```python
from build123d import *

# Parameters (mm, degrees)
F1_DEPTH      = 25.4
F1_DEPTH_BACK = 25.4
F2_W          = 25.4
F2_H          = 12.7
F3_DEPTH      = 12.7
F4_W          = 50.8
F4_H          = 12.7
F5_DEPTH      = 25.4
F6_W          = 25.4
F6_H          = 12.7
F7_DEPTH      = 12.7
F8_W          = 25.4
F8_H          = 12.7
F9_DEPTH      = 12.7
F10_R         = 6.35
F11_DEPTH     = 76.201
F13_DEPTH     = 12.701
F15_DEPTH     = 12.701


with BuildPart() as f1:
    # F0 (on Front) → F1 (new body, two sides)
    with BuildSketch(Plane.XZ) as f1_sk:
        Polygon((0, 38.1), (0, 0), (76.2, 0), (76.2, 12.7), (50.8, 12.7), (50.8, 25.4), (25.4, 25.4), (25.4, 50.8), (12.7, 50.8), align=None)
    extrude(amount=-F1_DEPTH)
    extrude(f1_sk.sketch, amount=F1_DEPTH_BACK)

    # F2 (on face) → F3 (join)
    with BuildSketch(Plane.YZ.offset(25.4)):
        with Locations((0, 44.45)):
            Rectangle(F2_W, F2_H)
    extrude(amount=F3_DEPTH)

    # F4 (on face) → F5 (join)
    with BuildSketch(Plane.YZ.offset(25.4)):
        with Locations((0, 31.75)):
            Rectangle(F4_W, F4_H)
    extrude(amount=F5_DEPTH)

    # F6 (on face) → F7 (cut)
    with BuildSketch(Plane.XZ.offset(25.4)):
        with Locations((38.1, 31.75)):
            Rectangle(F6_W, F6_H)
    extrude(amount=-F7_DEPTH, mode=Mode.SUBTRACT)

    # F8 (on face) → F9 (cut)
    with BuildSketch(Plane(origin=(0, 25.4, 0), x_dir=(-1, 0, 0), z_dir=(0, 1, 0))):
        with Locations((-38.1, 31.75)):
            Rectangle(F8_W, F8_H)
    extrude(amount=-F9_DEPTH, mode=Mode.SUBTRACT)

    # F10 (on face) → F11 (cut, through all)
    with BuildSketch(Plane.YZ.offset(76.2)):
        with Locations((0, 12.7)):
            Circle(F10_R)
    extrude(amount=-F11_DEPTH, mode=Mode.SUBTRACT)

    # F12 (on face) → F13 (cut, through all)
    with BuildSketch(Plane.XY.offset(12.7)):
        with BuildLine():
            Line((76.2, -25.4), (76.2, -15.875))
            ThreePointArc((76.2, -15.875), (71.6804078091, -22.740231571), (63.9032778758, -25.4))
            Line((63.9032778758, -25.4), (76.2, -25.4))
        make_face()
    extrude(amount=-F13_DEPTH, mode=Mode.SUBTRACT)

    # F14 (on face) → F15 (cut, through all)
    with BuildSketch(Plane.XY.offset(12.7)):
        with BuildLine():
            ThreePointArc((63.5, 25.4), (71.4375, 22.7541666667), (76.2, 15.875))
            Line((76.2, 15.875), (76.2, 25.4))
            Line((76.2, 25.4), (63.5, 25.4))
        make_face()
    extrude(amount=-F15_DEPTH, mode=Mode.SUBTRACT)


solid = f1.part
```
The listing builds one solid part. Answer for the finished solid, in the listing's coordinates (mm). A direction names the side the tool comes from. Give positions to 0.01 mm unless a question says otherwise; leave off trailing zeros. Order: outer loops, then holes, each group sorted by start corner. A loop starts at its lowest first (then second) coordinate and runs counter-clockwise, first axis right, second up. Notation, with made-up numbers: (71, 88.5) -> (129, 88.5) arc R21 ccw to (129, 93.5) -> close; hole circle Ø4 at (36.25, 68.5). An arc over 180 degrees is marked (long way). Write each question's results on one line, items separated by ' | '.
Q1. The part is cut by section A-A, the plane y = 0. Give the vertices of the cut face in (x, z).
Checked values:
outline: (0, 0) -> (76.2, 0) -> (76.2, 6.35) -> (0, 6.35) -> close; (0, 19.05) -> (50.8, 19.05) -> (50.8, 38.1) -> (38.1, 38.1) -> (38.1, 50.8) -> (12.7, 50.8) -> (0, 38.1) -> close
Q2. The part is cut by section B-B, the plane x = 33. Give the vertices of the cut face in (y, z).
Checked values:
outline: (-25.4, 0) -> (25.4, 0) -> (25.4, 25.4) -> (12.7, 25.4) -> (12.7, 50.8) -> (-12.7, 50.8) -> (-12.7, 25.4) -> (-25.4, 25.4) -> close; hole circle Ø12.7 at (0, 12.7)
Q3. Which of the six approach directions +Z, -Z, +X, -X, +Y, -Y give full straight-line access (tool end or side, diameter ignored) to faces 4 (the face through (35, 12.7, 35)), 5 (the face through (38, -19, 25.4)), 6 (the face through (71.342, 22.825, 6.439)), 7 (the face through (50.8, 0, 26))?
Checked values:
face 4: +Z, +X, +Y | face 5: +Z, +X, -Y | face 6: +Z, -Z, +X, +Y | face 7: +Z, +X, +Y, -Y
Q4. Determine the mould class of faces 1 (the face through (25.4, -19, 38)), 2 (the face through (30.167, 2.93, 7.066)), 3 (the face through (35, -12.7, 35)) for opening direction Y: pulls with the +Y half, pulls with the -Y half, needs draft (parallel to the pull), parting line crosses it, or undercut.
Checked values:
face 1: needs draft | face 2: undercut | face 3: pulls with the -Y half
Q5. Straight lines are drawn through the part: probe 1 along Z at (x, y) = (24, 0); probe 2 along Y at (x, z) = (22.5, 13); probe 3 along Z at (x, y) = (47.5, 15). For each, find the intervals that lie inside material, in ascending order. Write a range as from..to.
Checked values:
probe 1: z = 0..6.35, 19.05..50.8 | probe 2: y = -25.4..-6.34, 6.34..25.4 | probe 3: z = 0..25.4
Q6. The part is cut by section C-C, the plane y = -20. Give the vertices of the cut face in (x, z), and give its area (3 significant figures).
Checked values:
outline: (0, 0) -> (74.3, 0) -> (74.3, 12.7) -> (50.8, 12.7) -> (50.8, 25.4) -> (25.4, 25.4) -> (25.4, 50.8) -> (12.7, 50.8) -> (0, 38.1) -> close | area: 2,150 mm^2
Q7. The part is cut by section D-D, the plane z = 20. Give the vertices of the cut face in (x, y).
Checked values:
outline: (0, -25.4) -> (50.8, -25.4) -> (50.8, 25.4) -> (0, 25.4) -> close
Q8. Each of these flat-tipped pins is pushed along its axis until it touches: P1, Ø1, axis at y = -17.5, z = 43, coming from the +X side; P2, Ø10, axis at y = 1, z = 47, coming from the +X side; P3, Ø14, axis at x = 41.5, y = -19.5, coming from the +Z side; P4, Ø7.5, axis at y = 0, z = 12.7, coming from the +X side. Where does it stop, or does it pass through?
Checked values:
P1: stops at x = 25.4 | P2: stops at x = 38.1 | P3: stops at z = 38.1 | P4: passes through
